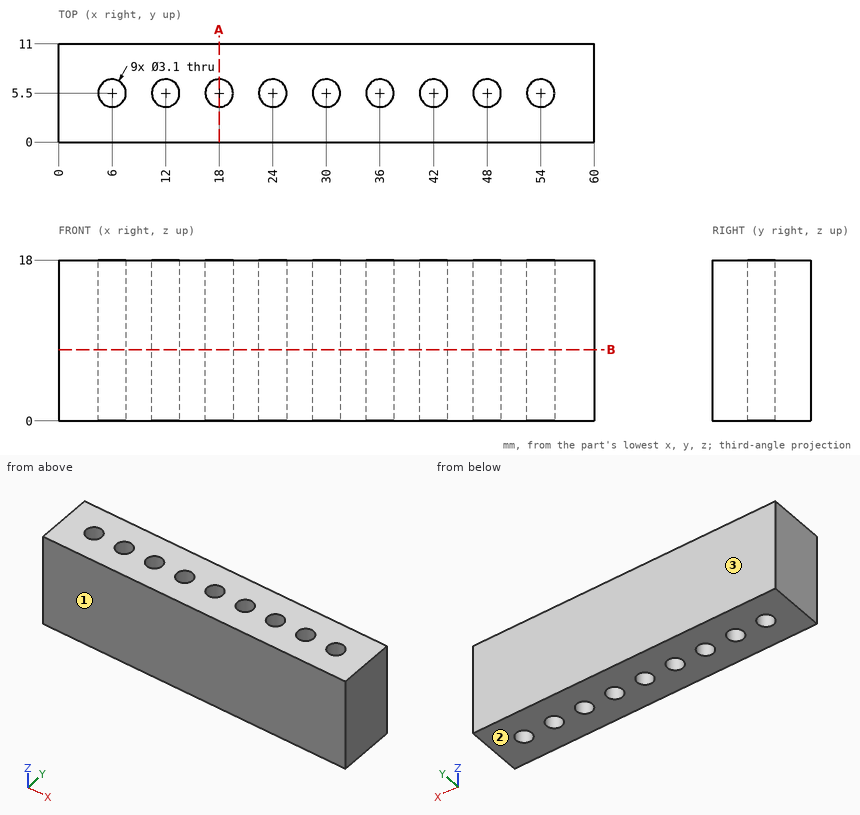
Input: dimensioned drawing with shaded views. Units: mm. Origin: part minimum x, y, z. Round coordinates to 2 decimals unless told otherwise and drop trailing zeros. Loops run counter-clockwise (first coordinate to the right, second up) from the corner with the lowest first, then second, coordinate; pieces in that order, holes last. Notation, with made-up numbers: M 11.5,85 L 44.5,85 A15 ccw 44.5,107 Z; hole C -22.5,86.5 d4. An arc over 180 degrees is marked long. One line per question, with ' | ' between items.
(1) Cut plane B-B on z = 8. Give the number of separate pieces and of enclosed holes in the cut face, plus the area to 3 significant figures.
Check result:
separate pieces: 1 | enclosed holes: 9 | area: 592 mm2
(2) Cut plane A-A on x = 18. Return the cut outline in (y, z).
Check result:
outline: M 0,0 L 3.95,0 L 3.95,18 L 0,18 Z; M 7.05,0 L 11,0 L 11,18 L 7.05,18 Z
(3) Pull-direction query (Y, two-part tool) for the marked faces 1, 2 and 3; classes: +Y half, -Y half, draft (parallel to the pull), parting line (faces both ways), or undercut.
Check result:
face 1: -Y half | face 2: draft | face 3: +Y half
(4) Material intervals for line 1 along Y through (x, z) = (24, 10.5); line 2 along Y through (x, z) = (43, 8.5), sorted ascending. Write a range as from..to.
Check result:
line 1: y = 0..3.95, 7.05..11 | line 2: y = 0..4.32, 6.68..11
(5) Contact query for flat-ended pins moving along their axis: P1, Ø8, axis at x = 38.5, z = 6, coming from the -Y side; P2, Ø3, axis at x = 36, y = 5.5, coming from the +Z side. Output: stop coordinate, or through.
Check result:
P1: stops at y = 0 | P2: passes through
